from build123d import *

# Parameters (mm, degrees)
CUT_EXTRUDE1_DEPTH       = 118.311258623
F_0_257_DIAMETER_HOLE1_D = 6.5278
CUT_EXTRUDE2_DEPTH       = 38.1


with BuildPart() as part:
    # Sketch2 → Revolve1 (revolve)
    with BuildSketch(Plane.XY, mode=Mode.PRIVATE) as revolve1_sk:
        Polygon((0, 0), (-25.4, 0), (-25.4, 39.67011582), (-48.421941822, 95.25), (-43.267048969, 95.25), (-22.225, 44.45), (-19.05, 44.45), (-19.05, 6.35), (0, 6.35), align=None)
    revolve(revolve1_sk.sketch.rotate(Axis((0, 0, 0), (0, -1, 0)), 270), axis=Axis((0, 0, 0), (0, -1, 0)))

    # Sketch3 → Cut-Extrude1 (cut, through all)
    with BuildSketch(Plane(origin=(0, 0, 0), x_dir=(0, 0, -1), z_dir=(1, 0, 0))):
        with BuildLine():
            Line((-3.81, 51.435), (-3.81, 13.335))
            ThreePointArc((-3.81, 13.335), (0, 9.525), (3.81, 13.335))
            Line((3.81, 13.335), (3.81, 51.435))
            ThreePointArc((3.81, 51.435), (0, 55.245), (-3.81, 51.435))
        make_face()
    extrude(amount=CUT_EXTRUDE1_DEPTH, mode=Mode.SUBTRACT)

    # F (0.257) Diameter Hole1 (through all)
    with Locations(Plane(origin=(0, 0, 0), x_dir=(-1, 0, 0), z_dir=(0, -1, 0))):
        with Locations((0, 0)):
            Hole(F_0_257_DIAMETER_HOLE1_D / 2)

    # Sketch8 → Cut-Extrude2 (cut, symmetric)
    with BuildSketch(Plane(origin=(0, 44.45, 0), x_dir=(1, 0, 0), z_dir=(0, 1, 0))):
        with BuildLine():
            Line((15.604846444, 10.926631112), (18.725815732, 13.111957335))
            ThreePointArc((18.725815732, 13.111957335), (22.86, 0), (18.725815732, -13.111957335))
            Line((18.725815732, -13.111957335), (15.604846444, -10.926631112))
            ThreePointArc((15.604846444, -10.926631112), (19.05, 0), (15.604846444, 10.926631112))
        make_face()
    extrude(amount=CUT_EXTRUDE2_DEPTH, both=True, mode=Mode.SUBTRACT)


solid = part.part
For this review, take the finished solid that the model builds, in its own axes (mm). A direction names the side the tool comes from. Round coordinates to 2 decimals unless told otherwise and drop trailing zeros. Loops run counter-clockwise (first coordinate to the right, second up) from the corner with the lowest first, then second, coordinate; pieces in that order, holes last. Notation, with made-up numbers: (28, -19) - (87, -19) arc R11 cw to (87, -15) - close; hole circle Ø11 at (44, 54). An arc over 180 degrees is marked (long way). Use one line per item in the form item = value.
Item 1: Consider section B-B on z = 0. Write out the cut boundary in (x, y) (3 decimals), then the cut area to 3 significant figures.
Answers:
outline = (-48.422, 95.25) - (-25.4, 39.67) - (-25.4, 0) - (-3.264, 0) - (-3.264, 6.35) - (-19.05, 6.35) - (-19.05, 44.45) - (-22.225, 44.45) - (-43.267, 95.25) - close; (3.264, 0) - (25.4, 0) - (25.4, 9.525) - (22.86, 9.525) - (22.86, 6.35) - (3.264, 6.35) - close; (26.696, 55.245) - (31.851, 55.245) - (48.422, 95.25) - (43.267, 95.25) - close
area = 1,000 mm^2
Item 2: Consider section A-A on x = 0. Write out the cut boundary in (y, z) (3 decimals).
Answers:
outline = (0, -25.4) - (39.67, -25.4) - (95.25, -48.422) - (95.25, -43.267) - (44.45, -22.225) - (44.45, -19.05) - (6.35, -19.05) - (6.35, -3.264) - (0, -3.264) - close; (0, 3.264) - (6.35, 3.264) - (6.35, 19.05) - (44.45, 19.05) - (44.45, 22.225) - (95.25, 43.267) - (95.25, 48.422) - (39.67, 25.4) - (0, 25.4) - close
Item 3: For line 1 (Y direction, x = 3, z = -5); line 2 (X direction, y = 53, z = 15); line 3 (Z direction, x = -17, y = 51.5), list the stretches that pass through material, from the lowest coordinate up.
Answers:
line_1 = 0 to 6.35
line_2 = -27.04 to -20.95, 20.95 to 27.04
line_3 = -25.08 to -18.53, 18.53 to 25.08
Item 4: Consider section D-D on y = 48. Write out the cut boundary in (x, z).
Answers:
outline = (23.39, -3.81) arc R23.7 cw (long way) to (23.39, 3.81) - (28.6, 3.81) arc R28.85 ccw (long way) to (28.6, -3.81) - close
Item 5: Mouldability with a two-part tool opening along Z and no side actions: class faces 4 (the conical face through (19.445, 55.498, -25.359)), 5 (the flat face through (0, 0, -5)), 6 (the flat face through (24.6, 36.4, -3.81)), 7 (the flat face through (2, 6.35, 4)) as +Z half, -Z half, draft (parallel to the pull), parting line (faces both ways), or undercut.
Answers:
face_4 = parting line
face_5 = draft
face_6 = undercut
face_7 = undercut
Item 6: Consider section C-C on y = 79. Write out the cut boundary in (x, z).
Answers:
outline = circle Ø83.38 at (0, 0); hole circle Ø73.07 at (0, 0)
Item 7: Tool access review of faces 1 (the flat face through (24.6, 36.9, 3.81)), 2 (the flat face through (-19, 44.45, -5)), 3 (the cylindrical face through (23.955, 9.526, 0.084)): name each direction out of +Z, -Z, +X, -X, +Y, -Y from which nothing blocks a thin tool from reaching the whole face with its end or side.
Answers:
face_1 = +X
face_2 = +Y
face_3 = +X, +Y
Item 8: Clearance check with flat-ended pins moving along their axes: P1, Ø2, axis at x = 24.5, y = 28.5, coming from the +Z side; P2, Ø2, axis at x = 17, y = 45.5, coming from the +Z side; P3, Ø8, axis at x = 26.5, y = 33.5, coming from the -Z side. State where each tip first meets the part, or that it passes through.
Answers:
P1 = 9.64
P2 = 22.92
P3 = -11.79
